```python
from build123d import *

# Parameters (mm, degrees)
F0_W     = 215.9
F0_H     = 271.78
F1_DEPTH = 17.78
F4_DEPTH = 7.62
F3_W     = 228.6
F3_H     = 279.4
F5_DEPTH = 7.62
F6_W     = 33.02
F6_H     = 279.043264
F7_DEPTH = 7.62


with BuildPart() as f1:
    # F0 (on Front) → F1 (new body)
    with BuildSketch(Plane.XZ):
        with Locations((27.200282, -20.502186)):
            Rectangle(F0_W, F0_H)
    extrude(amount=F1_DEPTH)

    # F2 (on face) → F4 (join)
    with BuildSketch(Plane.XZ.offset(17.78)):
        Polygon((147.850282, -160.202186), (147.850282, 119.197814), (-80.749718, 119.197814), (-80.749718, -159.84545), align=None)
    extrude(amount=F4_DEPTH)

    # F3 (on face) → F5 (join)
    with BuildSketch(Plane(origin=(0, 0, 0), x_dir=(-1, 0, 0), z_dir=(0, 1, 0))):
        with Locations((-33.550282, -20.502186)):
            Rectangle(F3_W, F3_H)
    extrude(amount=F5_DEPTH)

    # F6 (on face) → F7 (join)
    with BuildSketch(Plane(origin=(-80.749718, 0, 0), x_dir=(0, -1, 0), z_dir=(-1, 0, 0))):
        with Locations((8.89, -20.323818)):
            Rectangle(F6_W, F6_H)
    extrude(amount=F7_DEPTH)


solid = f1.part
```
Model file for the job. Use its own axes, mm. A direction names the side the tool comes from. Give positions to 0.01 mm unless a question says otherwise; leave off trailing zeros. Loops run counter-clockwise (first coordinate to the right, second up) from the corner with the lowest first, then second, coordinate; pieces in that order, holes last. Notation, with made-up numbers: (77, 21) - (108, 21) arc R26 cw to (108, 37) - close; hole circle Ø9 at (10.25, 81.25). An arc over 180 degrees is marked (long way). One line per item, written item: value. Start each with the question number.
1. Slice it at B-B (z = -76). List the corners of the cut face in (x, y), plus the area to 3 significant figures.
2. Pin check, flat tips, straight feed: pin 1 (1.1 mm diameter, centred on y = -9, z = 117, fed in from +X); pin 2 (4 mm diameter, centred on x = 58, y = -2.5, fed in from -Z); pin 3 (3 mm diameter, centred on y = -4.5, z = -157.5, fed in from +X). Stop position of each tip, or through.
3. Slice it at A-A (y = -4.5). List the corners of the cut face in (x, z).
4. Pull direction Y, two halves, no side cores. Call faces 1 (the flat face through (143, -17.78, -20)), 2 (the flat face through (31, 7.62, -22)), 3 (the flat face through (-88.37, -9, -18)): pulls with the +Y half, pulls with the -Y half, needs draft (parallel to the pull), parting line crosses it, or undercut.
5. Probe L1, parallel to Z at x = 129.5, y = -22.5; L2, parallel to Z at x = 38, y = -6.5; L3, parallel to X at y = -15, z = 83. List the from-to ranges inside material, lowest first. Write a range as from..to.
6. Which spindle directions (+Z, -Z, +X, -X, +Y, -Y) get a long thin tool onto all of the face, cutting with end or side? Do faces 4 (the flat face through (-85, -9, -159.845)), 5 (the flat face through (26, -9, 115.388)), 6 (the flat face through (135.15, -9, -22)). Say none if no direction does.
Solution:
1. outline: (-88.37, -25.4) - (147.85, -25.4) - (147.85, -17.78) - (135.15, -17.78) - (135.15, 0) - (147.85, 0) - (147.85, 7.62) - (-88.37, 7.62) - close
1. area: 7,570 mm^2
2. pin 1: stops at x = -80.75
2. pin 2: stops at z = -156.39
2. pin 3: stops at x = 135.15
3. outline: (-88.37, -159.85) - (-80.75, -159.85) - (-80.75, -156.39) - (135.15, -156.39) - (135.15, 115.39) - (-80.75, 115.39) - (-80.75, 119.2) - (-88.37, 119.2) - close
4. face 1: undercut
4. face 2: pulls with the +Y half
4. face 3: needs draft
5. L1: z = -160.17..119.2
5. L2: z = -156.39..115.39
5. L3: x = -88.37..135.15
6. face 4: -Z, -X, +Y, -Y
6. face 5: +Z, +X
6. face 6: +Z, -Z, +X
